Geometry: final body of the model. Coordinates: model frame, mm. A direction names the side the tool comes from. Coordinates: 2 decimals unless noted, no trailing zeros. Order: outer loops, then holes, each group sorted by start corner. A loop starts at its lowest first (then second) coordinate and runs counter-clockwise, first axis right, second up. Notation, with made-up numbers: M 53,69 L 71,69 A14 ccw 71,91 Z; hole C 42,47 d6. An arc over 180 degrees is marked long. Write item = value, one per line. Start each with the question number.
```python
from build123d import *

# Parameters (mm, degrees)
SKETCH1_R                = 19.939
CIRCLE_EXTRUDE_DEPTH     = 7.62
SKETCH3_W                = 7.62
SKETCH3_H                = 39.878
RECTANGLE_EXTRUDE_DEPTH  = 63.5
SKETCH2_R                = 18.034
CRICLE_CUT_DEPTH         = 67.991627245
EXTENSION_START          = 2.54
EXTENSION_DEPTH          = 2.54
SKETCH15_R               = 18.034
CIRCLE_CUT_2_DEPTH       = 67.991627245
SKETCH16_W               = 5.08
SKETCH16_H               = 39.878
MIDDLE_CUT_DEPTH         = 49.167836997
SKETCH18_W               = 5.08
SKETCH18_H               = 1.905
CUT_EXTRUDE5_DEPTH       = 17.78
SKETCH19_R               = 1.905
FOR_SPRING_EXTRUDE_DEPTH = 2.54


with BuildPart() as part:
    # Sketch1 → circle extrude (new body)
    with BuildSketch(Plane.XY):
        with Locations(Location((0, 0, 0), (0, 0, 180))):
            Circle(SKETCH1_R)
    extrude(amount=CIRCLE_EXTRUDE_DEPTH)

    # Sketch3 → rectangle extrude (add)
    with BuildSketch(Plane(origin=(0, 0, 0), x_dir=(0, 0, -1), z_dir=(1, 0, 0))):
        with Locations((-3.81, 0)):
            Rectangle(SKETCH3_W, SKETCH3_H)
    extrude(amount=RECTANGLE_EXTRUDE_DEPTH)

    # Sketch2 → cricle cut (cut, through all)
    with BuildSketch(Plane.XY.offset(7.62)):
        Circle(SKETCH2_R)
    extrude(amount=-CRICLE_CUT_DEPTH, mode=Mode.SUBTRACT)

    # Sketch10 → extension (add)
    with BuildSketch(Plane(origin=(0, 0, 0), x_dir=(-1, 0, 0), z_dir=(0, 0, -1)).offset(EXTENSION_START)):
        with BuildLine():
            Line((0, 19.939), (-63.5, 19.939))
            Line((-63.5, 19.939), (-63.5, -19.939))
            Line((-63.5, -19.939), (0, -19.939))
            ThreePointArc((0, -19.939), (19.939, 0), (0, 19.939))
        make_face()
    extrude(amount=-EXTENSION_DEPTH)

    # Sketch15 → circle cut 2 (cut, through all)
    with BuildSketch(Plane.XY):
        Circle(SKETCH15_R)
    extrude(amount=-CIRCLE_CUT_2_DEPTH, mode=Mode.SUBTRACT)

    # Sketch16 → middle cut (cut, through all)
    with BuildSketch(Plane(origin=(20.32, 0, 0), x_dir=(0, 0, -1), z_dir=(1, 0, 0))):
        with Locations((-2.54, 0)):
            Rectangle(SKETCH16_W, SKETCH16_H)
    extrude(amount=MIDDLE_CUT_DEPTH, mode=Mode.SUBTRACT)

    # Sketch18 → Cut-Extrude5 (cut)
    with BuildSketch(Plane(origin=(20.32, 0, 0), x_dir=(0, 0, -1), z_dir=(1, 0, 0))):
        with Locations((-2.54, 18.9865)):
            Rectangle(SKETCH18_W, SKETCH18_H)
    extrude(amount=-CUT_EXTRUDE5_DEPTH, mode=Mode.SUBTRACT)

    # Sketch19 → for spring extrude (add)
    with BuildSketch(Plane(origin=(20.32, 0, 0), x_dir=(0, 0, -1), z_dir=(1, 0, 0))):
        with Locations((-2.54, 0)):
            Circle(SKETCH19_R)
    extrude(amount=FOR_SPRING_EXTRUDE_DEPTH)


solid = part.part
```
Item 1: Draft query along X for faces 4 (the flat face through (22.86, 0, 3)), 5 (the cylindrical face through (-19.934, -0.438, 2.469)), 6 (the cylindrical face through (-3.909, -17.605, 2.611)). Return one class per face: pulls with the +X half, pulls with the -X half, needs draft (parallel to the pull), parting line crosses it, or undercut.
Item 2: Material intervals for probe 1 along Z at (x, y) = (47, 15); probe 2 along Y at (x, z) = (0, 4.5); probe 3 along X at (y, z) = (14, 3), sorted ascending. Write a range as [from, to].
Item 3: Reachability of faces 1 (the flat face through (20.32, -0.7, 4.8)), 2 (the flat face through (32, 0, -2.54)), 3 (the flat face through (2.54, 19, 3)) from +Z, -Z, +X, -X, +Y, -Y: full face, straight path, thin tool, end or side. Return the list, or none.
Item 4: Section query D-D on y = 9.5. Output: boundary loops of the cut face in (x, z), and give its area (3 significant figures).
Item 5: Section query C-C on z = 2.54. Output: boundary loops of the cut face in (x, y) (3 decimals), and give its area (3 significant figures).
Item 6: Section query B-B on y = 0. Output: boundary loops of the cut face in (x, z) (3 decimals).
Item 7: Section query A-A on x = 30. Output: boundary loops of the cut face in (y, z).
Item 8: First-contact query: pin 1 (1.5 mm diameter, centred on x = 8, z = 2.5, fed in from +Y); pin 2 (4 mm diameter, centred on y = 0.5, z = 2.5, fed in from +X); pin 3 (2.5 mm diameter, centred on y = 7, z = 2, fed in from +X); pin 4 (8 mm diameter, centred on x = -11, y = -13.5, fed in from -Z). Flat tips, straight axial feed; report the tip coordinate or a pass-through.
Ans:
q1.face_4 = pulls with the +X half
q1.face_5 = pulls with the -X half
q1.face_6 = undercut
q2.probe_1 = [-2.54, 0], [5.08, 7.62]
q2.probe_2 = [-19.94, -18.03], [18.03, 19.94]
q2.probe_3 = [-14.2, -11.37], [11.37, 20.32]
q3.face_1 = +X
q3.face_2 = -Z, +X, -X, +Y, -Y
q3.face_3 = +X, +Y
q4.outline = M -17.53,-2.54 L -15.33,-2.54 L -15.33,7.62 L -17.53,7.62 Z; M 15.33,-2.54 L 63.5,-2.54 L 63.5,0 L 20.32,0 L 20.32,5.08 L 63.5,5.08 L 63.5,7.62 L 15.33,7.62 Z
q4.area = 292 mm^2
q5.outline = M 0,-19.939 L 20.32,-19.939 L 20.32,-1.905 L 22.86,-1.905 L 22.86,1.905 L 20.32,1.905 L 20.32,18.034 L 2.54,18.034 L 2.54,19.939 L 0,19.939 A19.939 ccw Z; hole C 0,0 d36.068
q5.area = 389 mm^2
q6.outline = M -19.939,-2.54 L -18.034,-2.54 L -18.034,7.62 L -19.939,7.62 Z; M 18.034,-2.54 L 63.5,-2.54 L 63.5,0 L 20.32,0 L 20.32,0.635 L 22.86,0.635 L 22.86,4.445 L 20.32,4.445 L 20.32,5.08 L 63.5,5.08 L 63.5,7.62 L 18.034,7.62 Z
q7.outline = M -19.94,-2.54 L 19.94,-2.54 L 19.94,0 L -19.94,0 Z; M -19.94,5.08 L 19.94,5.08 L 19.94,7.62 L -19.94,7.62 Z
q8.pin_1 = 18.03
q8.pin_2 = 22.86
q8.pin_3 = 20.32
q8.pin_4 = -2.54
